The model under review builds one solid part; all positions refer to its coordinate system, in mm. A direction names the side the tool comes from. Round coordinates to 2 decimals unless told otherwise and drop trailing zeros. Loops run counter-clockwise (first coordinate to the right, second up) from the corner with the lowest first, then second, coordinate; pieces in that order, holes last. Notation, with made-up numbers: (-28.5, -4) -> (-11.5, -4) arc R30 cw to (-11.5, 27) -> close; hole circle Ø3 at (20, -14). An arc over 180 degrees is marked (long way). Write each question's results on one line, items separated by ' | '. Start each with the question number.
Item 1: Tool access review of faces 5 (the flat face through (11.062, 740, 42)), 6 (the flat face through (9.562, 740, 41)), 7 (the flat face through (212, 740, 16.633)): name each direction out of +Z, -Z, +X, -X, +Y, -Y from which nothing blocks a thin tool from reaching the whole face with its end or side.
Item 2: We need section B-B (y = 1395.5). Give the boundary of the cut face in (x, z), and give its area (3 significant figures).
Item 3: We need section A-A (z = 27). Give the boundary of the cut face in (x, y), and give its area (3 significant figures).
Item 4: For L1, parallel to X at y = 1292, z = 54.5; L2, parallel to X at y = 914.5, z = 25; L3, parallel to Z at x = 117, y = 1378, list the stretches that pass through material, from the lowest coordinate up. Write a range as from..to.
Item 5: Mouldability with a two-part tool opening along X and no side actions: class faces 1 (the flat face through (204.3, 1500, 17.7)), 2 (the flat face through (217, 740, 18.133)), 3 (the flat face through (418.062, 740, 41)), 4 (the flat face through (419.562, 740, 41)) as pulls with the +X half, pulls with the -X half, needs draft (parallel to the pull), parting line crosses it, or undercut.
Item 6: Clearance check with flat-ended pins moving along their axes: pin 1 Ø3 at (x, y) = (288, 1113.5) entering from +Z; pin 2 Ø1.2 at (x, y) = (-8, 982) entering from -Z; pin 3 Ø1.6 at (y, z) = (1300, 17.5) entering from -X; pin 4 Ø1.6 at (x, z) = (196.5, 17.5) entering from -Y. State where each tip first meets the part, or that it passes through.
Item 7: We need section C-C (x = 375.5). Give the boundary of the cut face in (y, z), and give its area (3 significant figures).
from build123d import *

# Parameters (mm, degrees)
F1_DEPTH = 1500
F2_W     = 20
F2_H     = 100
F3_DEPTH = 1.5


with BuildPart() as f1:
    # F0 (on Front) → F1 (new body)
    with BuildSketch(Plane.XZ):
        Polygon((9.56153, 65.133369), (9.56153, 16.633369), (419.56153, 16.633369), (419.56153, 65.133369), (403.56153, 65.133369), (403.56153, 63.633369), (418.06153, 63.633369), (418.06153, 18.133369), (11.06153, 18.133369), (11.06153, 66.633369), (-8.93847, 66.633369), (-8.93847, 51.633369), (-7.43847, 51.633369), (-7.43847, 65.133369), align=None)
    extrude(amount=-F1_DEPTH)

    # F2 (on face) → F3 (cut, through all)
    with BuildSketch(Plane.XY.offset(18.133369)):
        with Locations((198.56153, 182)):
            Rectangle(F2_W, F2_H)
        with Locations((198.56153, 1307)):
            Rectangle(F2_W, F2_H)
    extrude(amount=-F3_DEPTH, mode=Mode.SUBTRACT)


solid = f1.part
Here are the results:
1) face 5: +Z, +Y, -Y | face 6: -Z, +Y, -Y | face 7: -Z, +X, -X, +Y, -Y
2) outline: (-8.94, 51.63) -> (-7.44, 51.63) -> (-7.44, 65.13) -> (9.56, 65.13) -> (9.56, 16.63) -> (419.56, 16.63) -> (419.56, 65.13) -> (403.56, 65.13) -> (403.56, 63.63) -> (418.06, 63.63) -> (418.06, 18.13) -> (11.06, 18.13) -> (11.06, 66.63) -> (-8.94, 66.63) -> close | area: 828 mm2
3) outline: (9.56, 0) -> (11.06, 0) -> (11.06, 1500) -> (9.56, 1500) -> close; (418.06, 0) -> (419.56, 0) -> (419.56, 1500) -> (418.06, 1500) -> close | area: 4,500 mm2
4) L1: x = -8.94..-7.44, 9.56..11.06, 418.06..419.56 | L2: x = 9.56..11.06, 418.06..419.56 | L3: z = 16.63..18.13
5) face 1: needs draft | face 2: undercut | face 3: undercut | face 4: pulls with the +X half
6) pin 1: stops at z = 18.13 | pin 2: stops at z = 51.63 | pin 3: stops at x = 9.56 | pin 4: stops at y = 0
7) outline: (0, 16.63) -> (1500, 16.63) -> (1500, 18.13) -> (0, 18.13) -> close | area: 2,250 mm2
